```python
from build123d import *

# Parameters (mm, degrees)
SKETCH1_R           = 2.0193
SKETCH1_R_2         = 14.2875
BOSS_EXTRUDE1_DEPTH = 3.175
FILLET1_R           = 2.54


with BuildPart() as part:
    # Sketch1 → Boss-Extrude1 (new body)
    with BuildSketch(Plane(origin=(0, 0, 0), x_dir=(1, 0, 0), z_dir=(0, 1, 0))):
        with BuildLine():
            Line((11.158213086, 21.466758583), (-52.341786914, 21.466758583))
            Line((-52.341786914, 21.466758583), (-52.341786914, -29.333241417))
            add(Edge.make_bspline(
                [(-52.341786914, -29.333241417), (0, -31.75), (18.346437912, -12.413665165)],
                knots=[0, 0, 0, 1, 1, 1], degree=2))
            ThreePointArc((18.346437912, -12.413665165), (24.451434564, 6.58435381), (11.158213086, 21.466758583))
        make_face()
        with Locations((-39.641786914, -16.633241417)):
            Circle(SKETCH1_R, mode=Mode.SUBTRACT)
        with Locations((-39.641786914, -3.933241417)):
            Circle(SKETCH1_R, mode=Mode.SUBTRACT)
        with Locations((-39.641786914, 8.766758583)):
            Circle(SKETCH1_R, mode=Mode.SUBTRACT)
        with Locations((4.808213086, 2.416758583)):
            Circle(SKETCH1_R_2, mode=Mode.SUBTRACT)
    extrude(amount=BOSS_EXTRUDE1_DEPTH)

    # Fillet1
    fillet1_edges = [part.edges().sort_by_distance(p)[0] for p in [
        (-52.341786914, 1.5875, -21.466758583),
        (-52.341786914, 1.5875, 29.333241417),
    ]]
    fillet(fillet1_edges, radius=FILLET1_R)


solid = part.part
```
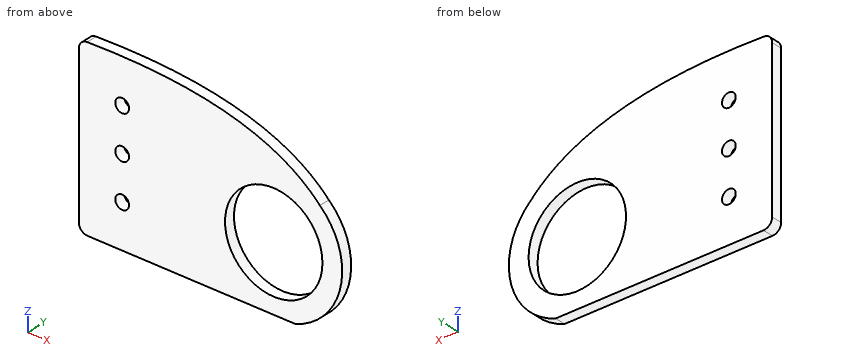
Here's how the part is built. I have some questions about the finished solid (model axes, mm). Round coordinates to 2 decimals unless told otherwise and drop trailing zeros. Order: outer loops, then holes, each group sorted by start corner. A loop starts at its lowest first (then second) coordinate and runs counter-clockwise, first axis right, second up. Notation, with made-up numbers: (13, -17.75) -> (55, -17.75) arc R12 cw to (55, -5.75) -> close; hole circle Ø5 at (-33.5, -4.5). An arc over 180 degrees is marked (long way). Use a Markdown table: item, result. Add a question column.
(1) Suppose I cut it at B-B, the plane y = 1.8. Count the separate pieces of the cut face and the enclosed holes in it, and give its area (3 significant figures).
(2) I need wall thicknesses on line 1 along X through (y, z) = (1.75, -7); line 2 along X through (y, z) = (0.45, -2); line 3 along X through (y, z) = (1.75, -12). Which ranges of each line are inside material? Lowest first, please.
(3) Suppose I cut it at C-C, the plane z = 0. Please give me the cut outline in (x, y) (3 decimals), and give its area (3 significant figures).
(4) Suppose I cut it at A-A, the plane z = -13. Please give me the cut outline in (x, y) (3 decimals).
Verdict:
| question | item | result |
|---|---|---|
| 1 | separate pieces | 1 |
| 1 | enclosed holes | 4 |
| 1 | area | 2,780 mm2 |
| 2 | line 1 | -52.34 to -40.62, -38.66 to -8.72, 18.34 to 24.36 |
| 2 | line 2 | -52.34 to -9.47, 19.09 to 24.88 |
| 2 | line 3 | -52.34 to -5.79, 15.41 to 22.45 |
| 3 | outline | (-52.342, 0) -> (-9.273, 0) -> (-9.273, 3.175) -> (-52.342, 3.175) -> close; (18.89, 0) -> (24.743, 0) -> (24.743, 3.175) -> (18.89, 3.175) -> close |
| 3 | area | 155 mm2 |
| 4 | outline | (-52.342, 0) -> (-4.79, 0) -> (-4.79, 3.175) -> (-52.342, 3.175) -> close; (14.407, 0) -> (21.873, 0) -> (21.873, 3.175) -> (14.407, 3.175) -> close |
